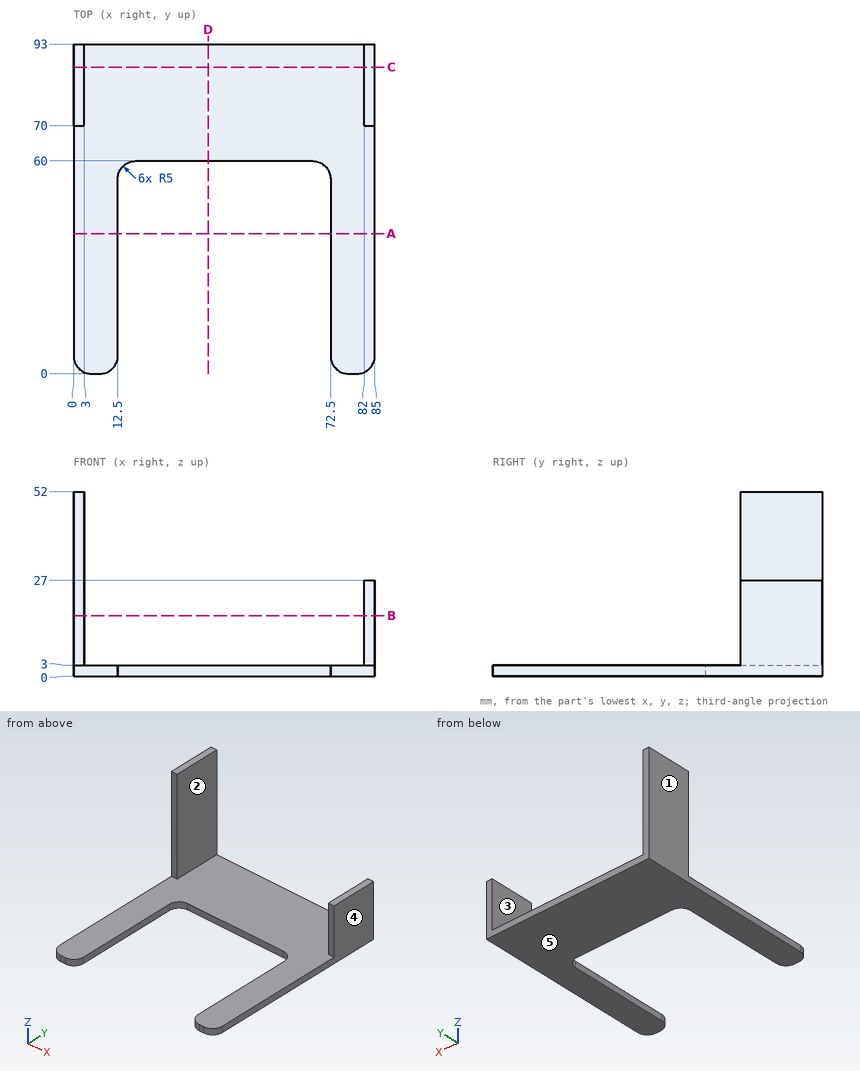
Geometry check sheet. Reference: drawing and pictorial views, mm from the part's lowest x, y, z. A direction names the side the tool comes from. Coordinates: 2 decimals unless noted, no trailing zeros. Write each loop counter-clockwise with the first axis right and the second up, starting at its lowest first coordinate (ties: lowest second). Pieces come first, ordered by that corner, then holes. Notation, with made-up numbers: M 21,47 L 66,47 A32 ccw 66,83 Z; hole C 84.5,-39.75 d9. An arc over 180 degrees is marked long. Write item = value, one per line. Start each with the question number.
1. Sectioned sample at B-B (z = 17). Record the cut outline in (x, y), then the cut area to 3 significant figures.
2. Mould release check, pull along X, two halves, no side actions. Record for the marked faces 3, 4 and 5: pulls with the +X half, pulls with the -X half, needs draft (parallel to the pull), parting line crosses it, or undercut.
3. Sectioned sample at D-D (x = 38). Record the cut outline in (y, z).
4. Sectioned sample at C-C (y = 86.5). Record the cut outline in (x, z), then the cut area to 3 significant figures.
5. Tool access check on the marked faces 1 and 2. Record the directions out of +Z, -Z, +X, -X, +Y, -Y that give a thin tool (end or side, any length) a straight path to the whole face; none if there is none.
6. Thickness scan on probe 1 along X at (y, z) = (78, 15); probe 2 along Z at (x, y) = (25, 72.5). Record the ranges inside material, lowest first.
7. Go/stop test with flat-tipped pins: pin 1 (10 mm diameter, centred on y = 65.5, z = 29.5, fed in from +X); pin 2 (3.5 mm diameter, centred on x = 53, z = 1, fed in from -Y); pin 3 (1 mm diameter, centred on x = 74, y = 69.5, fed in from +Z). Record where each tip stops, or that it passes through.
8. Sectioned sample at A-A (y = 39.5). Record the cut outline in (x, z).
The answers:
q1.outline = M 0,70 L 3,70 L 3,93 L 0,93 Z; M 82,70 L 85,70 L 85,93 L 82,93 Z
q1.area = 138 mm²
q2.face_3 = undercut
q2.face_4 = pulls with the +X half
q2.face_5 = needs draft
q3.outline = M 60,0 L 93,0 L 93,3 L 60,3 Z
q4.outline = M 0,0 L 85,0 L 85,27 L 82,27 L 82,3 L 3,3 L 3,52 L 0,52 Z
q4.area = 474 mm²
q5.face_1 = +Z, -Z, -X, +Y, -Y
q5.face_2 = +Z, +Y, -Y
q6.probe_1 = 0 to 3, 82 to 85
q6.probe_2 = 0 to 3
q7.pin_1 = 3
q7.pin_2 = 60
q7.pin_3 = 3
q8.outline = M 0,0 L 12.5,0 L 12.5,3 L 0,3 Z; M 72.5,0 L 85,0 L 85,3 L 72.5,3 Z
